```python
from build123d import *

# Parameters (mm, degrees)
BOSS_EXTRUDE1_DEPTH = 6
SKETCH5_W           = 200
SKETCH5_H           = 20
BOSS_EXTRUDE2_DEPTH = 6
SKETCH6_W           = 86.5
SKETCH6_H           = 143.586884574
BOSS_EXTRUDE3_DEPTH = 6
CUT_EXTRUDE3_DEPTH  = 230.888016217
CUT_EXTRUDE4_DEPTH  = 228.130469114
SKETCH9_W           = 210
SKETCH9_H           = 52
CUT_EXTRUDE5_DEPTH  = 226.140511681
BOSS_EXTRUDE4_DEPTH = 6
FILLET1_R           = 10
SKETCH11_R          = 1.3
CUT_EXTRUDE6_DEPTH  = 259.163707751
SKETCH12_R          = 1.3
CUT_EXTRUDE7_DEPTH  = 259.163707751
SKETCH13_R          = 1.75
CUT_EXTRUDE8_DEPTH  = 10
CUT_EXTRUDE9_DEPTH  = 259.163707751
SKETCH15_R          = 208.652698437
CUT_EXTRUDE10_DEPTH = 259.163707751


with BuildPart() as part:
    # Sketch2 → Boss-Extrude1 (new body)
    with BuildSketch(Plane(origin=(0, 0, 0), x_dir=(1, 0, 0), z_dir=(0, 1, 0))):
        with BuildLine():
            Line((-100, -128.086884574), (-100, 35.5))
            Line((-100, 35.5), (100, 35.5))
            Line((100, 35.5), (100, -128.086884574))
            ThreePointArc((100, -128.086884574), (0, 162.5), (-100, -128.086884574))
        make_face()
    extrude(amount=BOSS_EXTRUDE1_DEPTH)

    # Sketch5 → Boss-Extrude2 (add)
    with BuildSketch(Plane(origin=(0, 6, 0), x_dir=(1, 0, 0), z_dir=(0, 1, 0))):
        with Locations((0, -118.086884574)):
            Rectangle(SKETCH5_W, SKETCH5_H)
    extrude(amount=-BOSS_EXTRUDE2_DEPTH)

    # Sketch6 → Boss-Extrude3 (add, through all)
    with BuildSketch(Plane(origin=(0, 6, 0), x_dir=(1, 0, 0), z_dir=(0, 1, 0))):
        with Locations((-56.75, -36.293442287)):
            Rectangle(SKETCH6_W, SKETCH6_H)
        with Locations((56.75, -36.293442287)):
            Rectangle(SKETCH6_W, SKETCH6_H)
    extrude(amount=-BOSS_EXTRUDE3_DEPTH)

    # Sketch7 → Cut-Extrude3 (cut, through all)
    with BuildSketch(Plane(origin=(0, 6, 0), x_dir=(1, 0, 0), z_dir=(0, 1, 0))):
        with BuildLine():
            Line((-150, -62.5), (-100, -62.5))
            Line((-100, -62.5), (-100, 35.5))
            Line((-100, 35.5), (-158.574903437, 35.5))
            ThreePointArc((-158.574903437, 35.5), (-161.881492944, -14.164471125), (-150, -62.5))
        make_face()
        with BuildLine():
            Line((100, 35.5), (100, -62.5))
            Line((100, -62.5), (150, -62.5))
            ThreePointArc((150, -62.5), (161.881492944, -14.164471125), (158.574903437, 35.5))
            Line((158.574903437, 35.5), (100, 35.5))
        make_face()
    extrude(amount=-CUT_EXTRUDE3_DEPTH, mode=Mode.SUBTRACT)

    # Sketch8 → Cut-Extrude4 (cut, through all)
    with BuildSketch(Plane(origin=(0, 6, 0), x_dir=(1, 0, 0), z_dir=(0, 1, 0))):
        with BuildLine():
            Line((-30, 132.5), (-30, 159.706762537))
            ThreePointArc((-30, 159.706762537), (0, 162.5), (30, 159.706762537))
            Line((30, 159.706762537), (30, 132.5))
            ThreePointArc((30, 132.5), (0, 102.5), (-30, 132.5))
        make_face()
    extrude(amount=-CUT_EXTRUDE4_DEPTH, mode=Mode.SUBTRACT)

    # Sketch9 → Cut-Extrude5 (cut, through all)
    with BuildSketch(Plane(origin=(0, 6, 0), x_dir=(1, 0, 0), z_dir=(0, 1, 0))):
        with Locations((0, 81)):
            Rectangle(SKETCH9_W, SKETCH9_H)
    extrude(amount=-CUT_EXTRUDE5_DEPTH, mode=Mode.SUBTRACT)

    # Sketch10 → Boss-Extrude4 (add, through all)
    with BuildSketch(Plane(origin=(0, 6, 0), x_dir=(1, 0, 0), z_dir=(0, 1, 0))):
        with BuildLine():
            Line((-100, -128.086884574), (-130, -128.086884574))
            ThreePointArc((-130, -128.086884574), (0, 182.5), (130, -128.086884574))
            Line((130, -128.086884574), (100, -128.086884574))
            ThreePointArc((100, -128.086884574), (0, 162.5), (-100, -128.086884574))
        make_face()
    extrude(amount=-BOSS_EXTRUDE4_DEPTH)

    # Fillet1
    fillet1_edges = [part.edges().sort_by_distance(p)[0] for p in [
        (-105, 3, -107),
        (105, 3, -107),
        (105, 3, -55),
        (-105, 3, -55),
    ]]
    fillet(fillet1_edges, radius=FILLET1_R)

    # Sketch11 → Cut-Extrude6 (cut, through all)
    with BuildSketch(Plane(origin=(0, 6, 0), x_dir=(1, 0, 0), z_dir=(0, 1, 0))):
        with Locations(Location((0, 177.5, 0), (0, 0, 270))):
            Circle(SKETCH11_R)
        with Locations(Location((88.75, 153.719509172, 0), (0, 0, 270))):
            Circle(SKETCH11_R)
        with Locations(Location((153.719509172, 88.75, 0), (0, 0, 270))):
            Circle(SKETCH11_R)
        with Locations(Location((177.5, 0, 0), (0, 0, 270))):
            Circle(SKETCH11_R)
        with Locations(Location((153.719509172, -88.75, 0), (0, 0, 270))):
            Circle(SKETCH11_R)
        with Locations((88.75, -153.719509172)):
            Circle(SKETCH11_R)
        with Locations((0, -177.5)):
            Circle(SKETCH11_R)
        with Locations((-88.75, -153.719509172)):
            Circle(SKETCH11_R)
        with Locations(Location((-153.719509172, -88.75, 0), (0, 0, 270))):
            Circle(SKETCH11_R)
        with Locations(Location((-177.5, 0, 0), (0, 0, 270))):
            Circle(SKETCH11_R)
        with Locations(Location((-153.719509172, 88.75, 0), (0, 0, 270))):
            Circle(SKETCH11_R)
        with Locations(Location((-88.75, 153.719509172, 0), (0, 0, 270))):
            Circle(SKETCH11_R)
    extrude(amount=-CUT_EXTRUDE6_DEPTH, mode=Mode.SUBTRACT)

    # Sketch12 → Cut-Extrude7 (cut, through all)
    with BuildSketch(Plane(origin=(0, 6, 0), x_dir=(1, 0, 0), z_dir=(0, 1, 0))):
        with Locations(Location((0, -118.086884574, 0), (0, 0, 270))):
            Circle(SKETCH12_R)
        with Locations(Location((-90, -118.086884574, 0), (0, 0, 270))):
            Circle(SKETCH12_R)
        with Locations(Location((90, -118.086884574, 0), (0, 0, 270))):
            Circle(SKETCH12_R)
        with Locations(Location((-90, 25.5, 0), (0, 0, 270))):
            Circle(SKETCH12_R)
        with Locations(Location((-90, -41.293442287, 0), (0, 0, 270))):
            Circle(SKETCH12_R)
        with Locations(Location((90, -41.293442287, 0), (0, 0, 90))):
            Circle(SKETCH12_R)
        with Locations(Location((90, 25.5, 0), (0, 0, 90))):
            Circle(SKETCH12_R)
    extrude(amount=-CUT_EXTRUDE7_DEPTH, mode=Mode.SUBTRACT)

    # Sketch13 → Cut-Extrude8 (cut)
    with BuildSketch(Plane(origin=(0, 6, 0), x_dir=(1, 0, 0), z_dir=(0, 1, 0))):
        with Locations(Location((-17.875, -13.5, 0), (0, 0, 270))):
            Circle(SKETCH13_R)
        with Locations(Location((17.875, -13.5, 0), (0, 0, 270))):
            Circle(SKETCH13_R)
    extrude(amount=-CUT_EXTRUDE8_DEPTH, mode=Mode.SUBTRACT)

    # Sketch14 → Cut-Extrude9 (cut, through all)
    with BuildSketch(Plane(origin=(0, 6, 0), x_dir=(1, 0, 0), z_dir=(0, 1, 0))):
        with BuildLine():
            Line((-30, 132.5), (30, 132.5))
            ThreePointArc((30, 132.5), (37.46877708, 114.46877708), (55.5, 107))
            Line((55.5, 107), (-55.5, 107))
            ThreePointArc((-55.5, 107), (-37.46877708, 114.46877708), (-30, 132.5))
        make_face()
    extrude(amount=-CUT_EXTRUDE9_DEPTH, mode=Mode.SUBTRACT)

    # Sketch15 → Cut-Extrude10 (cut, through all)
    with BuildSketch(Plane(origin=(0, 6, 0), x_dir=(1, 0, 0), z_dir=(0, 1, 0))):
        Circle(SKETCH15_R)
        with BuildLine():
            Line((-95, 55), (-174.015085553, 55))
            ThreePointArc((-174.015085553, 55), (-177.444343068, -42.658587802), (-130, -128.086884574))
            Line((-130, -128.086884574), (-83, -128.086884574))
            Line((-83, -128.086884574), (-83, 55))
            Line((-83, 55), (-95, 55))
        make_face(mode=Mode.SUBTRACT)
    extrude(amount=-CUT_EXTRUDE10_DEPTH, mode=Mode.SUBTRACT)


solid = part.part
```
Can you work these out from the model? Positions are in its coordinate system, mm. A direction names the side the tool comes from. Give positions to 0.01 mm unless a question says otherwise; leave off trailing zeros. Loops run counter-clockwise (first coordinate to the right, second up) from the corner with the lowest first, then second, coordinate; pieces in that order, holes last. Notation, with made-up numbers: M -24,19.25 L -4,19.25 A17 ccw -4,40.25 Z; hole C 14.25,56 d9. An arc over 180 degrees is marked long. One line per item, written item: value.
(1) Suppose I cut it at B-B on y = 2.25. List the corners of the cut face in (x, z) for me.
Returned:
outline: M -174.02,-55 L -83,-55 L -83,128.09 L -130,128.09 A182.5 ccw Z; hole C -177.5,0 d2.6; hole M -158.57,-35.5 L -100,-35.5 L -100,62.5 L -150,62.5 A162.5 ccw Z; hole C -153.72,88.75 d2.6; hole C -90,-25.5 d2.6; hole C -90,41.29 d2.6; hole C -90,118.09 d2.6
(2) I need wall thicknesses on line 1 (X direction, y = 2.4, z = 0); line 2 (Z direction, x = -90, y = 4.05); line 3 (Z direction, x = -120, y = 3.7). Which ranges of each line are inside material? Lowest first, please.
Returned:
line 1: -182.5 to -178.8, -176.2 to -162.5, -100 to -83
line 2: -55 to -26.8, -24.2 to 39.99, 42.59 to 116.79, 119.39 to 128.09
line 3: -55 to -35.5, 62.5 to 128.09
(3) Will this pin go through, and if not, where does the flat tip stop? pin 1 (4 mm diameter, centred on x = -90, z = 41.29, fed in from +Y).
Returned:
pin 1: y = 6
(4) We'd pull the mould along X, two halves only. Please class faces 1 (the face through (-161.94, 3.04, 13.47)), 2 (the face through (-99, 6, 35)), 3 (the face through (-177.116, 3.042, 44.004)): released by +X, released by -X, zero draft, split by the parting line, or undercut.
Returned:
face 1: undercut
face 2: zero draft
face 3: released by -X
(5) Suppose I cut it at A-A on z = 49. List the corners of the cut face in (x, y) for me.
Returned:
outline: M -175.8,0 L -154.94,0 L -154.94,6 L -175.8,6 Z; M -100,0 L -83,0 L -83,6 L -100,6 Z
(6) Suppose I cut it at C-C on x = -140.5. List the corners of the cut face in (y, z) for me.
Returned:
outline: M 0,-55 L 6,-55 L 6,-35.5 L 0,-35.5 Z; M 0,62.5 L 6,62.5 L 6,116.47 L 0,116.47 Z
(7) Suppose I cut it at D-D on z = 102.5. List the corners of the cut face in (x, y) for me.
Returned:
outline: M -151,0 L -83,0 L -83,6 L -151,6 Z
(8) Which directions (+Z, -Z, +X, -X, +Y, -Y) give clear straight access to the entire face, cutting with the end or side of a thin tool? Please do faces 4 (the face through (-83, 3, 38)), 5 (the face through (-125, 3, 62.5)).
Returned:
face 4: +Z, -Z, +X, +Y, -Y
face 5: +Y, -Y
